```python
from build123d import *

# Parameters (mm, degrees)
F1_DEPTH = 3.175
F3_D     = 3.175


with BuildPart() as f1:
    # F0 (on Front) → F1 (new body)
    with BuildSketch(Plane.XZ):
        with BuildLine():
            Line((23.241043, -5.801166), (23.117982, -5.77672))
            ThreePointArc((23.117982, -5.77672), (23.179482, -5.789095), (23.241043, -5.801166))
        make_face()
        with BuildLine():
            Line((-24.51433, 3.685497), (23.117982, -5.77672))
            Line((23.117982, -5.77672), (23.241043, -5.801166))
            ThreePointArc((23.241043, -5.801166), (38.354, 6.6675), (23.241043, 19.136167))
            Line((23.241043, 19.136167), (23.117982, 19.11172))
            Line((23.117982, 19.11172), (-24.51433, 9.649503))
            ThreePointArc((-24.51433, 9.649503), (-28.194172, 6.6675), (-24.51433, 3.685497))
        make_face()
        with BuildLine():
            Line((23.117982, 19.11172), (23.241043, 19.136167))
            ThreePointArc((23.241043, 19.136167), (23.179482, 19.124095), (23.117982, 19.11172))
        make_face()
    extrude(amount=F1_DEPTH)

    # F3 (through all)
    with Locations(Plane.XZ.offset(3.175)):
        with Locations((-25.146, 6.6675)):
            Hole(F3_D / 2)


solid = f1.part
```
Could you check a few things on this model? Use its own coordinates, in mm. Coordinates: 2 decimals unless noted, no trailing zeros. Order: outer loops, then holes, each group sorted by start corner. A loop starts at its lowest first (then second) coordinate and runs counter-clockwise, first axis right, second up. Notation, with made-up numbers: M 13.25,13.5 L 69.25,13.5 A15 cw 69.25,21.5 Z; hole C 84.25,-37.75 d5. An arc over 180 degrees is marked long. Use a Markdown table: item, result. Add a question column.
Q1. I want a section at A-A on z = 7.25. List the corners of the cut face in (x, y) for me (3 decimals).
Q2. We'd pull the mould along X, two halves only. Please class faces 1 (the flat face through (12, -3.175, 7)), 2 (the cylindrical face through (-23.56, -1.57, 6.74)): pulls with the +X half, pulls with the -X half, needs draft (parallel to the pull), parting line crosses it, or undercut.
Q3. I want a section at C-C on x = -5. List the corners of the cut face in (y, z) for me (3 decimals), then the cut area to 3 significant figures.
Q4. I want a section at D-D on z = 12.5. List the corners of the cut face in (x, y) for me (3 decimals).
Q5. If I drill on L1, parallel to X at y = -1.1, z = 6.25; L2, parallel to Z at x = 33, y = -0.6; L3, parallel to Z at x = 31, y = -0.3, over which ranges is the centre line in solid material (lowest first)?
Checked values:
| question | item | result |
|---|---|---|
| 1 | outline | M -28.138,-3.175 L -26.623,-3.175 L -26.623,0 L -28.138,0 Z; M -23.669,-3.175 L 38.341,-3.175 L 38.341,0 L -23.669,0 Z |
| 2 | face 1 | needs draft |
| 2 | face 2 | undercut |
| 3 | outline | M -3.175,-0.191 L 0,-0.191 L 0,13.526 L -3.175,13.526 Z |
| 3 | area | 43.6 mm² |
| 4 | outline | M -10.165,-3.175 L 36.935,-3.175 L 36.935,0 L -10.165,0 Z |
| 5 | L1 | -28.17 to -26.68, -23.61 to 38.35 |
| 5 | L2 | -3.69 to 17.03 |
| 5 | L3 | -4.85 to 18.19 |
